from build123d import *

# Parameters (mm, degrees)
BASEHEAD_DEPTH = 13
SKETCH4_W      = 0.8
SKETCH4_H      = 3.629909152
HEADFILLET_R   = 1.2


with BuildPart() as part:
    # HeadSke → BaseHead (new body)
    with BuildSketch(Plane(origin=(0, 0, 0), x_dir=(0, 0, -1), z_dir=(1, 0, 0))):
        Polygon((17, 9.814954576), (17, -9.814954576), (0, -19.629909152), (-17, -9.814954576), (-17, 9.814954576), (0, 19.629909152), align=None)
    extrude(amount=BASEHEAD_DEPTH)

    # BodySke → BaseBody (revolve)
    with BuildSketch(Plane.XY, mode=Mode.PRIVATE) as basebody_sk:
        Polygon((0, 10.5), (0, 0), (138, 0), (138, 8.626), (136.626, 10), (112, 10), (110.133974596, 10.5), align=None)
    revolve(basebody_sk.sketch.rotate(Axis((0, 0, 0), (1, 0, 0)), 90), axis=Axis((0, 0, 0), (1, 0, 0)))

    # Sketch3 → HeadChamfer (revolve, cut)
    with BuildSketch(Plane(origin=(0, 0, 0), x_dir=(1, 0, 0), z_dir=(0, 1, 0))):
        Polygon((4.25, 24.361215932), (-4.25, 9.638784068), (-11.424013371, 13.780702619), (-2.924013371, 28.503134483), align=None)
    revolve(axis=Axis((0, 0, 0), (1, 0, 0)), mode=Mode.SUBTRACT)

    # Sketch4 → BearingFace (revolve, cut)
    with BuildSketch(Plane.XY, mode=Mode.PRIVATE) as bearingface_sk:
        with Locations((12.6, 17.814954576)):
            Rectangle(SKETCH4_W, SKETCH4_H)
    revolve(bearingface_sk.sketch.rotate(Axis((0, 0, 0), (1, 0, 0)), 90), axis=Axis((0, 0, 0), (1, 0, 0)), mode=Mode.SUBTRACT)

    # HeadFillet
    headfillet_edges = [part.edges().sort_by_distance(p)[0] for p in [
        (13, 0, -10.5),
    ]]
    fillet(headfillet_edges, radius=HEADFILLET_R)


solid = part.part
Here's how the part is built. I have some questions about the finished solid (model axes, mm). A direction names the side the tool comes from. Give positions to 0.01 mm unless a question says otherwise; leave off trailing zeros. Order: outer loops, then holes, each group sorted by start corner. A loop starts at its lowest first (then second) coordinate and runs counter-clockwise, first axis right, second up. Notation, with made-up numbers: M 29.25,17.25 L 67.25,17.25 A17 cw 67.25,49.25 Z; hole C -1,12 d10. An arc over 180 degrees is marked long. Answer as a JSON object with one key per item and string values. Group by question number.
1) On a 3-axis mill with a long thin cutter (end or side, diameter ignored), from which of +Z, -Z, +X, -X, +Y, -Y can I reach the whole of each face in a straight line? I mean faces 1 (the flat face through (12.2, 16, 3)), 2 (the flat face through (6.015, 14.654, 8.619)). Say none if no direction works.
2) I'm going to push flat-ended pins straight in: pin 1 Ø5 at (x, z) = (18.5, -7) entering from -Y; pin 2 Ø2 at (y, z) = (1, 9) entering from -X; pin 3 Ø5 at (x, y) = (42, -7) entering from +Z; pin 4 Ø12 at (x, y) = (100.5, 8) entering from +Z. Where does each tip first touch, or does it pass through?
3) Please list where these lines run through material, in increasing order: L1, parallel to X at y = 3, z = 15; L2, parallel to X at y = 16.5, z = -0.5; L3, parallel to Y at x = 65, z = -2.5. Write a range as [from, to].
4) Suppose I cut it at A-A, the plane x = 102. Write out the boundary of the cut face in (y, z), plus the area to 3 significant figures.
Results found:
{
 "1": {"face 1": "+X", "face 2": "+Z, +X, -X, +Y"},
 "2": {"pin 1": "y = -9.49", "pin 2": "x = 0", "pin 3": "z = 9.49", "pin 4": "z = 10.31"},
 "3": {"L1": "[0, 13]", "L2": "[0, 12.2]", "L3": "[-10.2, 10.2]"},
 "4": {"outline": "C 0,0 d21", "area": "346 mm²"}
}
